from build123d import *

# Parameters (mm, degrees)
SKETCH_R      = 12.5
SKETCH_R_2    = 1.5
PAD_DEPTH     = 3
SKETCH001_R   = 14.5
SKETCH001_R_2 = 12.5
PAD001_DEPTH  = 20


with BuildPart() as part:
    # Sketch → Pad (new body)
    with BuildSketch(Plane.XY):
        with BuildLine():
            ThreePointArc((-13.973189, 15), (0, -20.5), (13.973189, 15))
            Line((-13.973189, 15), (13.973189, 15))
        make_face()
        Circle(SKETCH_R, mode=Mode.SUBTRACT)
        with Locations((-17, 0)):
            Circle(SKETCH_R_2, mode=Mode.SUBTRACT)
        with Locations((17, 0)):
            Circle(SKETCH_R_2, mode=Mode.SUBTRACT)
    extrude(amount=PAD_DEPTH)

    # Sketch001 → Pad001 (new body)
    with BuildSketch(Plane.XY.offset(3)):
        Circle(SKETCH001_R)
        Circle(SKETCH001_R_2, mode=Mode.SUBTRACT)
    extrude(amount=PAD001_DEPTH)


solid = part.part
Could you check a few things on this model? Use its own coordinates, in mm. A direction names the side the tool comes from. Give positions to 0.01 mm unless a question says otherwise; leave off trailing zeros. Order: outer loops, then holes, each group sorted by start corner. A loop starts at its lowest first (then second) coordinate and runs counter-clockwise, first axis right, second up. Notation, with made-up numbers: (55.5, 27) - (71.5, 27) arc R28 cw to (71.5, 64) - close; hole circle Ø4 at (43.25, 62). An arc over 180 degrees is marked (long way). One line per question, with ' | ' between items. Start each with the question number.
Item 1: For faces 4 (the flat face through (4.3, -14.3, 3)), 5 (the cylindrical face through (-18.5, 0.07, 1.48)), which set-ups out of +Z, -Z, +X, -X, +Y, -Y let a thin tool reach every point of the face, with its end or its side?
Item 2: I want a section at A-A on x = 0. Write out the boundary of the cut face in (y, z), then the cut area to 4 significant figures.
Item 3: I want a section at C-C on z = 2.5. Write out the boundary of the cut face in (x, y), then the cut area to 3 significant figures.
Item 4: I'm going to push flat-ended pins straight in: pin 1 Ø1.5 at (y, z) = (-14, 7) entering from +X; pin 2 Ø12 at (y, z) = (-1, 16) entering from -X; pin 3 Ø5 at (x, z) = (-15, 9) entering from +Y; pin 4 Ø10.5 at (x, y) = (-3, -4) entering from +Z. Where does each tip first touch, or does it pass through?
Item 5: Thinking about a two-plate mould opening in Z: for faces 1 (the cylindrical face through (11.923, 3.755, 11.339)), 2 (the flat face through (9, -10, 0)), 3 (the flat face through (-11, 7, 23)), which applies, pulls with the +Z half, pulls with the -Z half, needs draft (parallel to the pull), parting line crosses it, or undercut?
Item 6: I need wall thicknesses on probe 1 along Y at (x, z) = (0, 4); probe 2 along Z at (x, y) = (12, -11); probe 3 along X at (y, z) = (-3.5, 4.5). Which ranges of each line are inside material? Lowest first, please. Write a range as [from, to].
Item 7: I want a section at D-D on y = 9. Write out the boundary of the cut face in (x, z).
Item 8: I want a section at B-B on y = 0. Write out the boundary of the cut face in (x, z).
Verdict:
1) face 4: +Z | face 5: +Z, -Z
2) outline: (-20.5, 0) - (-12.5, 0) - (-12.5, 23) - (-14.5, 23) - (-14.5, 3) - (-20.5, 3) - close; (12.5, 0) - (15, 0) - (15, 3) - (14.5, 3) - (14.5, 23) - (12.5, 23) - close | area: 111.5 mm^2
3) outline: (-13.97, 15) arc R20.5 ccw (long way) to (13.97, 15) - close; hole circle Ø3 at (-17, 0); hole circle Ø25 at (0, 0); hole circle Ø3 at (17, 0) | area: 710 mm^2
4) pin 1: x = 5.89 | pin 2: x = -14.5 | pin 3: y = 7.35 | pin 4: through
5) face 1: needs draft | face 2: pulls with the -Z half | face 3: pulls with the +Z half
6) probe 1: [-14.5, -12.5], [12.5, 14.5] | probe 2: [0, 3] | probe 3: [-14.07, -12], [12, 14.07]
7) outline: (-18.42, 0) - (-8.67, 0) - (-8.67, 23) - (-11.37, 23) - (-11.37, 3) - (-18.42, 3) - close; (8.67, 0) - (18.42, 0) - (18.42, 3) - (11.37, 3) - (11.37, 23) - (8.67, 23) - close
8) outline: (-20.5, 0) - (-18.5, 0) - (-18.5, 3) - (-20.5, 3) - close; (-15.5, 0) - (-12.5, 0) - (-12.5, 23) - (-14.5, 23) - (-14.5, 3) - (-15.5, 3) - close; (12.5, 0) - (15.5, 0) - (15.5, 3) - (14.5, 3) - (14.5, 23) - (12.5, 23) - close; (18.5, 0) - (20.5, 0) - (20.5, 3) - (18.5, 3) - close
